from build123d import *

# Parameters (mm, degrees)
F0_W     = 50
F0_H     = 150
F0_R     = 2.5
F0_W_2   = 20
F0_H_2   = 80
F1_DEPTH = 10
F2_DEPTH = 100
F4_DEPTH = 20
F5_W     = 10
F5_H     = 95
F6_DEPTH = 115.001
F7_R     = 1.5
F8_R     = 4
F9_DEPTH = 35.001
F10_SIZE = 1
F11_R    = 30
F12_R    = 3


with BuildPart() as f1:
    # F0 (on Top) → F1 (new body)
    with BuildSketch(Plane.XY):
        Rectangle(F0_W, F0_H)
        with Locations((0, -55)):
            Circle(F0_R, mode=Mode.SUBTRACT)
        Rectangle(F0_W_2, F0_H_2, mode=Mode.SUBTRACT)
        with Locations((0, 55)):
            Circle(F0_R, mode=Mode.SUBTRACT)
        Rectangle(F0_W_2, F0_H_2)
    extrude(amount=-F1_DEPTH)

    # F0 (on Top) → F2 (join)
    with BuildSketch(Plane.XY):
        Rectangle(F0_W_2, F0_H_2)
    extrude(amount=F2_DEPTH)

    # F3 (on face) → F4 (cut, through all)
    with BuildSketch(Plane(origin=(-10, 0, 0), x_dir=(0, -1, 0), z_dir=(-1, 0, 0))):
        with BuildLine():
            Line((-6, 100), (-6, 70))
            ThreePointArc((-6, 70), (0, 64), (6, 70))
            Line((6, 70), (6, 100))
            Line((6, 100), (-6, 100))
        make_face()
    extrude(amount=-F4_DEPTH, mode=Mode.SUBTRACT)

    # F5 (on face) → F6 (cut, through all)
    with BuildSketch(Plane.XZ.offset(40)):
        with Locations((0, 52.5)):
            Rectangle(F5_W, F5_H)
    extrude(amount=-F6_DEPTH, mode=Mode.SUBTRACT)

    # F7
    f7_edges = [f1.edges().sort_by_distance(p)[0] for p in [
        (5, 0, 5),
        (-5, 0, 5),
    ]]
    fillet(f7_edges, radius=F7_R)

    # F8 (on face) → F9 (cut, through all)
    with BuildSketch(Plane(origin=(-10, 0, 0), x_dir=(0, -1, 0), z_dir=(-1, 0, 0))):
        with Locations((0, 57)):
            Circle(F8_R)
    extrude(amount=-F9_DEPTH, mode=Mode.SUBTRACT)

    # F10
    f10_edges = [f1.edges().sort_by_distance(p)[0] for p in [
        (-10, 4, 57),
        (-5, 4, 57),
        (5, 4, 57),
        (10, 4, 57),
    ]]
    chamfer(f10_edges, length=F10_SIZE)

    # F11
    f11_edges = [f1.edges().sort_by_distance(p)[0] for p in [
        (-7.5, 40, 100),
        (7.5, 40, 100),
        (7.5, -40, 100),
        (-7.5, -40, 100),
    ]]
    fillet(f11_edges, radius=F11_R)

    # F12
    f12_edges = [f1.edges().sort_by_distance(p)[0] for p in [
        (-10, 31.213203, 91.213203),
        (-10, 8, 100),
        (-10, -8, 100),
        (-10, -31.213203, 91.213203),
        (10, -31.213203, 91.213203),
        (10, -8, 100),
        (10, 8, 100),
        (10, 31.213203, 91.213203),
    ]]
    fillet(f12_edges, radius=F12_R)


solid = f1.part
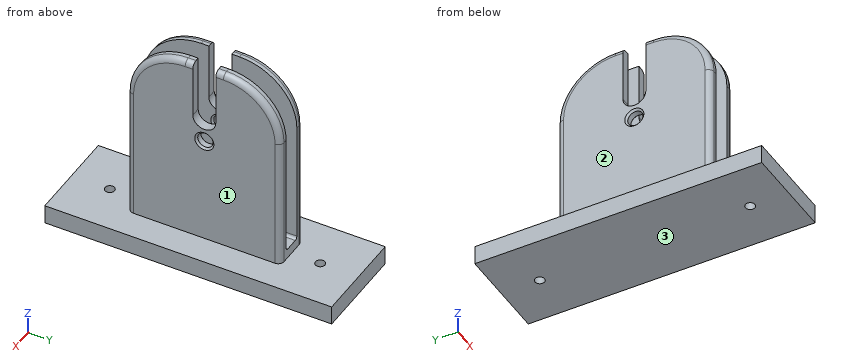
Source: CAD feature listing. Evaluate the final solid. Frame: model axes, mm. Face numbers are marked on the shaded views. A direction names the side the tool comes from. Round coordinates to 2 decimals unless told otherwise and drop trailing zeros. Loops run counter-clockwise (first coordinate to the right, second up) from the corner with the lowest first, then second, coordinate; pieces in that order, holes last.
Q1. First-contact query: P1, Ø1.5, axis at x = -6.5, z = 17, coming from the -Y side; P2, Ø4, axis at x = -7.5, z = 88, coming from the -Y side; P3, Ø2, axis at y = 50.5, z = 1.5, coming from the +X side; P4, Ø8, axis at x = 17.5, y = -2.5, coming from the +Z side. Flat tips, straight axial feed; report the tip coordinate or a pass-through.
Q2. Access query for the marked faces 1, 2 and 3. Directions: +Z, -Z, +X, -X, +Y, -Y. A direction counts if a zero-diameter tool reaches every point of the face in a straight line with its end or side. Return the directions, or none.
Q3. Ray query, line 1 (Y direction, x = 0, z = -5.75); line 2 (X direction, y = -22, z = 35); line 3 (Z direction, x = 7, y = 0). Return the intervals inside material, ascending.
Q4. Section D-D, the plane z = 44. Return loops of the section in (x, y).
Q5. Section A-A, the plane y = -55. Return loops of the section in (x, z), plus the area to 3 significant figures.
Q6. Section C-C, the plane x = 0. Return loops of the section in (y, z).
Q7. Section B-B, the plane z = 57. Return loops of the section in (x, y).
Solutions:
1. P1: stops at y = -40
1. P2: stops at y = -35.36
1. P3: passes through
1. P4: stops at z = 0
2. face 1: +Z, +X, +Y, -Y
2. face 2: +Z, -X, +Y, -Y
2. face 3: -Z, +X, -X, +Y, -Y
3. line 1: y = -75 to -57.5, -52.5 to 52.5, 57.5 to 75
3. line 2: x = -10 to -5, 5 to 10
3. line 3: z = -10 to 53, 61 to 64
4. outline: (-10, -37) arc R3 ccw to (-7, -40) - (-5, -40) - (-5, 40) - (-7, 40) arc R3 ccw to (-10, 37) - close; (5, -40) - (7, -40) arc R3 ccw to (10, -37) - (10, 37) arc R3 ccw to (7, 40) - (5, 40) - close
5. outline: (-25, -10) - (-2.5, -10) - (-2.5, 0) - (-25, 0) - close; (2.5, -10) - (25, -10) - (25, 0) - (2.5, 0) - close
5. area: 450 mm2
6. outline: (-75, -10) - (-57.5, -10) - (-57.5, 0) - (-75, 0) - close; (-52.5, -10) - (52.5, -10) - (52.5, 0) - (40, 0) - (40, 5) - (-40, 5) - (-40, 0) - (-52.5, 0) - close; (57.5, -10) - (75, -10) - (75, 0) - (57.5, 0) - close
7. outline: (-10, -37) arc R3 ccw to (-7, -40) - (-5, -40) - (-5, -5) - (-6, -4) - (-9, -4) - (-10, -5) - close; (-10, 5) - (-9, 4) - (-6, 4) - (-5, 5) - (-5, 40) - (-7, 40) arc R3 ccw to (-10, 37) - close; (5, -40) - (7, -40) arc R3 ccw to (10, -37) - (10, -5) - (9, -4) - (6, -4) - (5, -5) - close; (5, 5) - (6, 4) - (9, 4) - (10, 5) - (10, 37) arc R3 ccw to (7, 40) - (5, 40) - close
